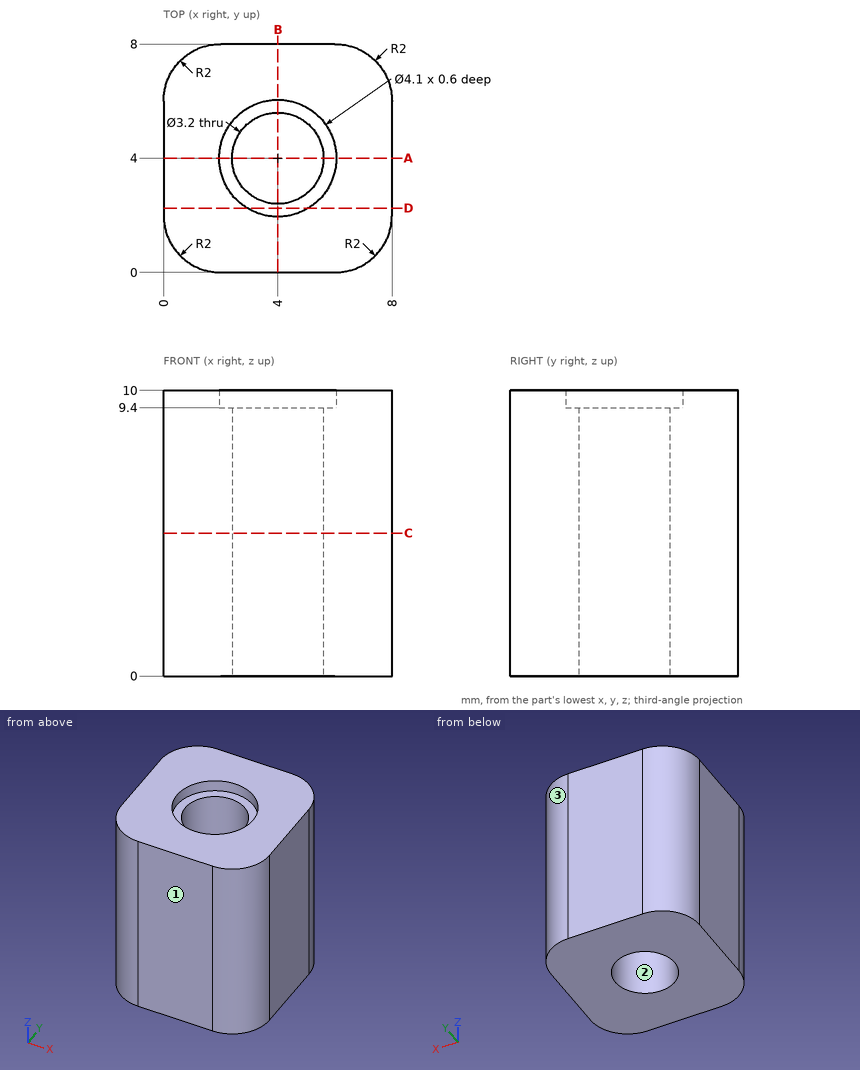
Input: dimensioned drawing with shaded views. Units: mm. Origin: part minimum x, y, z. Give positions to 0.01 mm unless a question says otherwise; leave off trailing zeros. Write each loop counter-clockwise with the first axis right and the second up, starting at its lowest first coordinate (ties: lowest second). Pieces come first, ordered by that corner, then holes.
1. Section query A-A (y = 4). Return the cut outline in (x, z).
2. Section query C-C (z = 5). Return the cut outline in (x, y).
3. Section query D-D (y = 2.25). Return the cut outline in (x, z), then the cut area to 3 significant figures.
4. Pull-direction query (X, two-part tool) for the marked faces 1, 2 and 3; classes: +X half, -X half, draft (parallel to the pull), parting line (faces both ways), or undercut.
5. Material intervals for line 1 along X through (y, z) = (4, 6); line 2 along X through (y, z) = (4, 9.85), sorted ascending.
6. First-contact query: pin 1 (2 mm diameter, centred on x = 4.5, y = 5, fed in from +Z). Flat tip, straight axial feed; report the tip coordinate or a pass-through.
Output values:
1. outline: (0, 0) - (2.4, 0) - (2.4, 9.4) - (1.95, 9.4) - (1.95, 10) - (0, 10) - close; (5.6, 0) - (8, 0) - (8, 10) - (6.05, 10) - (6.05, 9.4) - (5.6, 9.4) - close
2. outline: (0, 2) arc R2 ccw to (2, 0) - (6, 0) arc R2 ccw to (8, 2) - (8, 6) arc R2 ccw to (6, 8) - (2, 8) arc R2 ccw to (0, 6) - close; hole circle Ø3.2 at (4, 4)
3. outline: (0, 0) - (8, 0) - (8, 10) - (5.07, 10) - (5.07, 9.4) - (2.93, 9.4) - (2.93, 10) - (0, 10) - close
3. area: 78.7 mm2
4. face 1: draft
4. face 2: undercut
4. face 3: +X half
5. line 1: x = 0 to 2.4, 5.6 to 8
5. line 2: x = 0 to 1.95, 6.05 to 8
6. pin 1: stops at z = 10
